The figure shows three views and two pictorial views of one solid part (mm, origin at its lowest corner). Answer the questions. Coordinates: 2 decimals unless noted, no trailing zeros. Order: outer loops, then holes, each group sorted by start corner. A loop starts at its lowest first (then second) coordinate and runs counter-clockwise, first axis right, second up. Notation, with made-up numbers: (-10, -27.75) - (31, -27.75) arc R5 ccw to (31, -19.75) - close; hole circle Ø1 at (-1.5, 77.25). An arc over 180 degrees is marked (long way). Use one line per item in the form item = value.
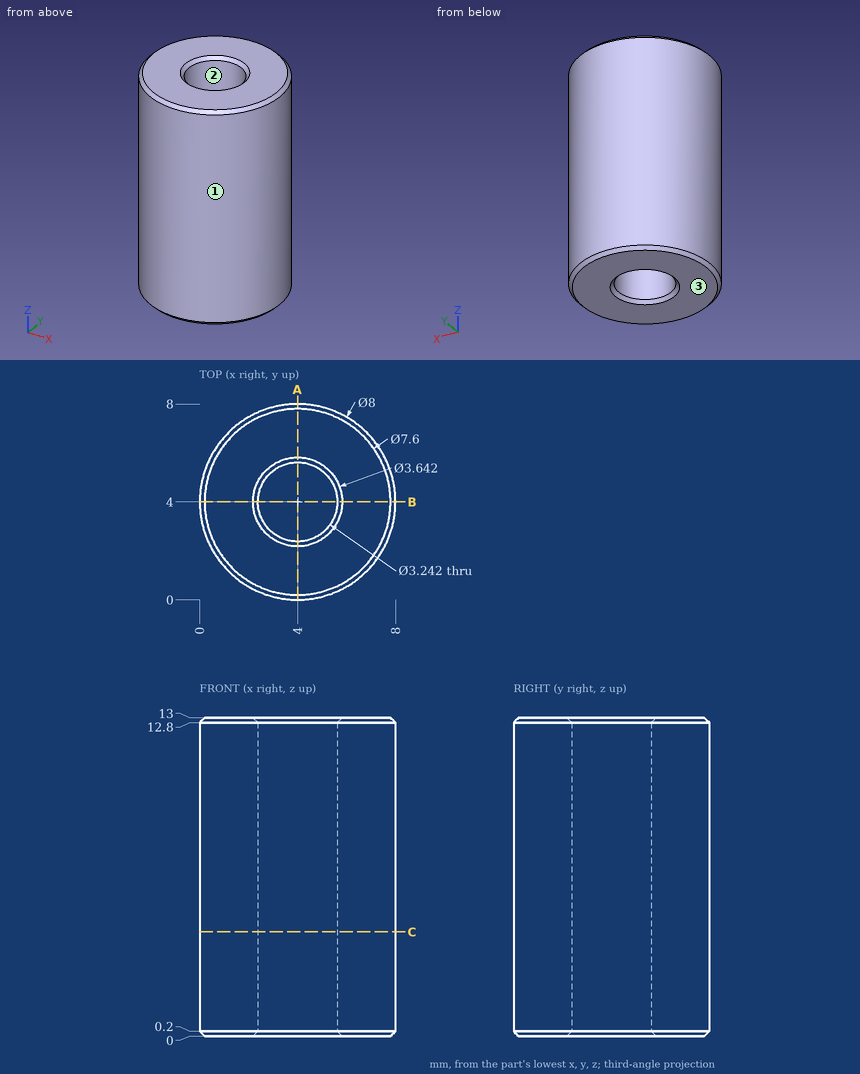
(1) Section C-C, the plane z = 4.25 is taken. Write down the section's boundary in (x, y).
Answer list:
outline = circle Ø8 at (4, 4); hole circle Ø3.24 at (4, 4)
(2) The mould has two halves that part along X. Classify the marked faces 1, 2 and 3: +X half, -X half, draft (parallel to the pull), parting line (faces both ways), or undercut.
Answer list:
face_1 = parting line
face_2 = undercut
face_3 = draft
(3) Section A-A, the plane x = 4 is taken. Write down the section's boundary in (y, z).
Answer list:
outline = (0, 0.2) - (0.2, 0) - (2.18, 0) - (2.38, 0.2) - (2.38, 12.8) - (2.18, 13) - (0.2, 13) - (0, 12.8) - close; (5.62, 0.2) - (5.82, 0) - (7.8, 0) - (8, 0.2) - (8, 12.8) - (7.8, 13) - (5.82, 13) - (5.62, 12.8) - close
(4) Straight lines are drawn through the part: L1, parallel to Y at x = 4, z = 5.5; L2, parallel to X at y = 3.5, z = 2.5. For each, find the intervals that lie inside material, in ascending order.
Answer list:
L1 = 0 to 2.38, 5.62 to 8
L2 = 0.03 to 2.46, 5.54 to 7.97
